```python
from build123d import *

# Parameters (mm, degrees)
F0_R     = 51.2202453394
F2_DEPTH = 25.4
F3_R     = 7.3585229381
F0_R_2   = 57.5702453394
F4_DEPTH = 6.604
F5_R     = 5.08


# Not quite as in the source:
# - the program builds the solid bodies; features that only make, move or delete a surface that nothing else refers to are left out


with BuildPart() as f2:
    # F0 (on Top) → F2 (new body)
    with BuildSketch(Plane.XY):
        Circle(F0_R)
    extrude(amount=F2_DEPTH)

    # F3
    f3_edges = [f2.edges().sort_by_distance(p)[0] for p in [
        (-51.220245, 0, 25.4),
    ]]
    fillet(f3_edges, radius=F3_R)

    # F0 (on Top) → F4 (join)
    with BuildSketch(Plane.XY):
        Circle(F0_R_2)
        Circle(F0_R, mode=Mode.SUBTRACT)
    extrude(amount=F4_DEPTH)

    # F5
    f5_edges = [f2.edges().sort_by_distance(p)[0] for p in [
        (-57.570245, 0, 6.604),
    ]]
    fillet(f5_edges, radius=F5_R)


solid = f2.part
```
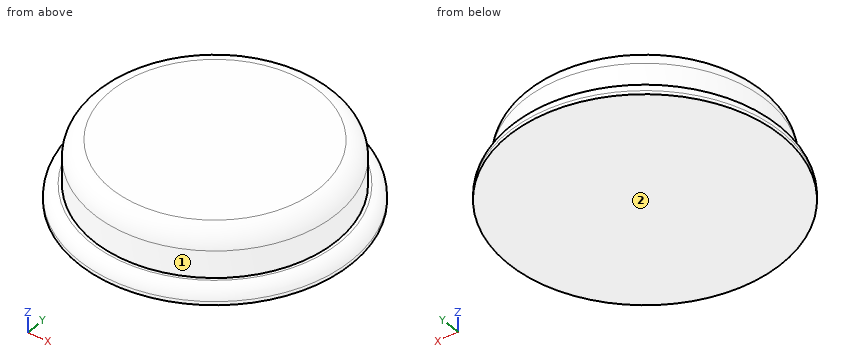
Can you work these out from the model? Positions are in its coordinate system, mm. Face numbers are marked on the shaded views. A direction names the side the tool comes from. Coordinates: 2 decimals unless noted, no trailing zeros. Loops run counter-clockwise (first coordinate to the right, second up) from the corner with the lowest first, then second, coordinate; pieces in that order, holes last.
1) For pin 1 (4 mm diameter, centred on x = 36, z = 10.5, fed in from -Y); pin 2 (12 mm diameter, centred on x = -40, z = 13, fed in from +Y); pin 3 (1 mm diameter, centred on x = 13, z = 13, fed in from +Y), each with a flat end and sliding along its axis, tell me the tip position at first contact or that it passes through.
2) Imagine slicing it at C-C on z = 14.25. List the corners of the cut face in (x, y) for me.
3) I need wall thicknesses on probe 1 along X at (y, z) = (27, 6.75); probe 2 along Y at (x, z) = (-19, 24); probe 3 along Y at (x, z) = (-13.5, 10.5). Which ranges of each line are inside material? Lowest first, please.
4) Imagine slicing it at D-D on z = 20.75. List the corners of the cut face in (x, y) for me, plus the area to 3 significant figures.
5) Imagine slicing it at A-A on y = 0. List the corners of the cut face in (x, z) for me, plus the area to 3 significant figures.
6) Which directions (+Z, -Z, +X, -X, +Y, -Y) give clear straight access to the entire face, cutting with the end or side of a thin tool? Please do the marked faces 1 and 2.
Completed:
1. pin 1: stops at y = -38.31
1. pin 2: stops at y = 38.31
1. pin 3: stops at y = 49.67
2. outline: circle Ø102.44 at (0, 0)
3. probe 1: x = -43.53 to 43.53
3. probe 2: y = -44.27 to 44.27
3. probe 3: y = -49.41 to 49.41
4. outline: circle Ø101.41 at (0, 0)
4. area: 8,080 mm2
5. outline: (-57.57, 0) - (57.57, 0) - (57.57, 1.52) arc R5.08 ccw to (52.49, 6.6) - (51.22, 6.6) - (51.22, 18.04) arc R7.36 ccw to (43.86, 25.4) - (-43.86, 25.4) arc R7.36 ccw to (-51.22, 18.04) - (-51.22, 6.6) - (-52.49, 6.6) arc R5.08 ccw to (-57.57, 1.52) - close
5. area: 2,650 mm2
6. face 1: +Z
6. face 2: -Z, +X, -X, +Y, -Y
